Input: dimensioned drawing with shaded views. Units: mm. Origin: part minimum x, y, z. A direction names the side the tool comes from. Round coordinates to 2 decimals unless told otherwise and drop trailing zeros. Order: outer loops, then holes, each group sorted by start corner. A loop starts at its lowest first (then second) coordinate and runs counter-clockwise, first axis right, second up. Notation, with made-up numbers: M 53.25,-37 L 108.25,-37 A13 ccw 108.25,-28 Z; hole C 30,13.25 d5. An arc over 180 degrees is marked long. Use CSV: the item, a comma, the result in double quotes. Start each with the question number.
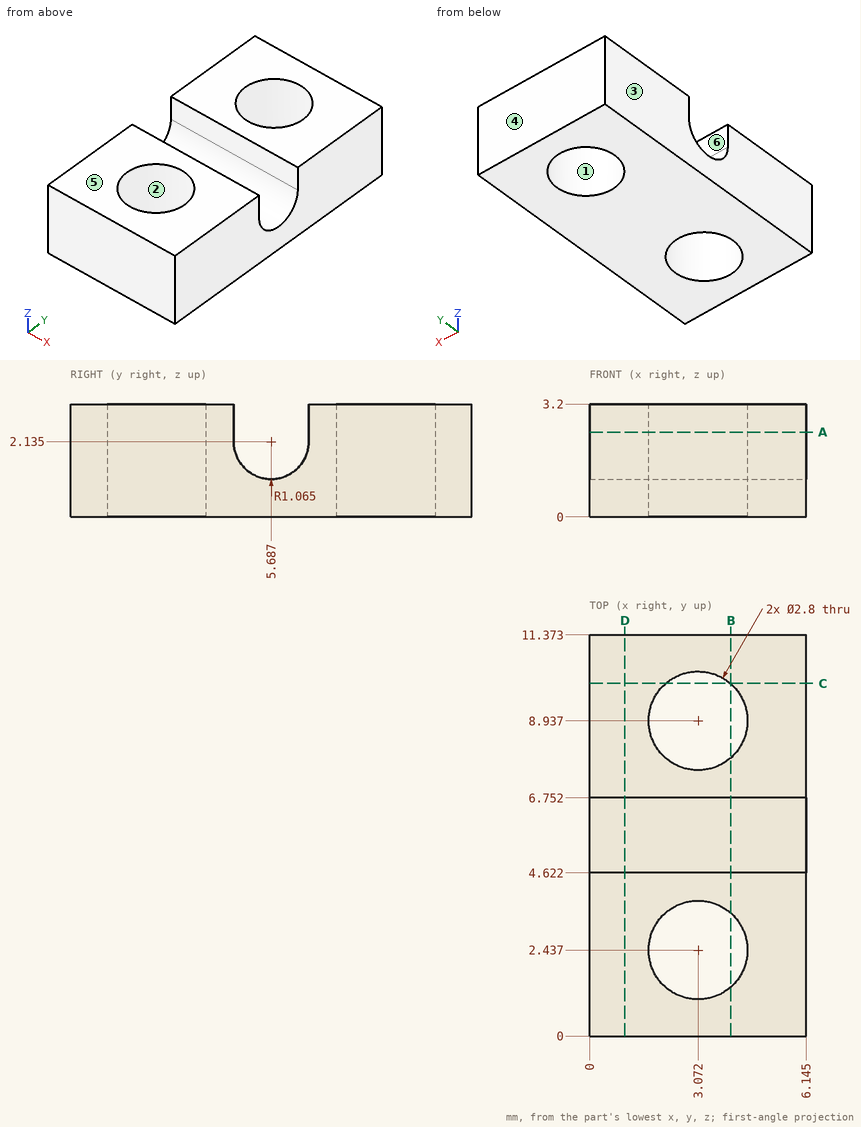
(1) Line query: line 1 along Y through (x, z) = (4, 0.5) (1 decimal); line 2 along Y through (x, z) = (5, 2.95); line 3 along Y through (x, z) = (2.75, 2.7) (1 decimal). Output: solid intervals per line, ascending.
(2) Section C-C on y = 10. Return loops of the section in (x, z) (1 decimal).
(3) Draft query along X for the marked faces 1, 2, 3 and 4. Return one class per face: pulls with the +X half, pulls with the -X half, needs draft (parallel to the pull), parting line crosses it, or undercut.
(4) Section B-B on x = 4. Return loops of the section in (y, z) (1 decimal).
(5) Section A-A on z = 2.4. Return loops of the section in (x, y) (1 decimal).
(6) Reachability of the marked faces 5 and 6 from +Z, -Z, +X, -X, +Y, -Y: full face, straight path, thin tool, end or side. Return the list, or none.
(7) Section D-D on x = 1. Return loops of the section in (y, z) (1 decimal).
Results below:
1,line 1,"y = 0 to 1.4, 3.5 to 7.9, 10 to 11.4"
1,line 2,"y = 0 to 4.62, 6.75 to 11.37"
1,line 3,"y = 0 to 1.1, 3.8 to 4.6, 6.8 to 7.6, 10.3 to 11.4"
2,outline,"M 0,0 L 2.2,0 L 2.2,3.2 L 0,3.2 Z; M 4,0 L 6.1,0 L 6.1,3.2 L 4,3.2 Z"
3,face 1,"undercut"
3,face 2,"undercut"
3,face 3,"pulls with the -X half"
3,face 4,"needs draft"
4,outline,"M 0,0 L 1.4,0 L 1.4,3.2 L 0,3.2 Z; M 3.5,0 L 7.9,0 L 7.9,3.2 L 6.8,3.2 L 6.8,2.1 A1.1 cw 4.6,2.1 L 4.6,3.2 L 3.5,3.2 Z; M 10,0 L 11.4,0 L 11.4,3.2 L 10,3.2 Z"
5,outline,"M 0,0 L 6.1,0 L 6.1,4.6 L 0,4.6 Z; M 0,6.8 L 6.1,6.8 L 6.1,11.4 L 0,11.4 Z; hole C 3.1,2.4 d2.8; hole C 3.1,8.9 d2.8"
6,face 5,"+Z, +X, -X, +Y, -Y"
6,face 6,"+Z, +X, -X"
7,outline,"M 0,0 L 11.4,0 L 11.4,3.2 L 6.8,3.2 L 6.8,2.1 A1.1 cw 4.6,2.1 L 4.6,3.2 L 0,3.2 Z"
